```python
from build123d import *

# Parameters (mm, degrees)
F1_DEPTH = 19.05
F2_W     = 128.431639
F2_H     = 61.237093
F3_DEPTH = 6.35
F4_R     = 15.24


with BuildPart() as f1:
    # F0 (on Top) → F1 (new body)
    with BuildSketch(Plane.XY):
        Polygon((-110.641599, 45.212001), (-110.641599, -23.367999), (26.518401, -23.367999), (26.518401, -16.519178), (-99.390604, -16.519178), (-99.390604, 38.352568), (26.518401, 38.352568), (26.518401, 45.212001), align=None)
    extrude(amount=F1_DEPTH)

    # F2 (on Top) → F3 (join)
    with BuildSketch(Plane.XY):
        with Locations((-37.725527, 10.113819)):
            Rectangle(F2_W, F2_H)
    extrude(amount=F3_DEPTH)

    # F4
    f4_edges = [f1.edges().sort_by_distance(p)[0] for p in [
        (-110.641599, 10.922001, 0),
    ]]
    fillet(f4_edges, radius=F4_R)


solid = f1.part
```
Part model, mm, in its own coordinate system. A direction names the side the tool comes from. Give positions to 0.01 mm unless a question says otherwise; leave off trailing zeros. Order: outer loops, then holes, each group sorted by start corner. A loop starts at its lowest first (then second) coordinate and runs counter-clockwise, first axis right, second up. Notation, with made-up numbers: (4.5, 39.25) - (37.5, 39.25) arc R20 ccw to (37.5, 78.25) - close; hole circle Ø5 at (-22, 71). An arc over 180 degrees is marked (long way). Use one line per item in the form item = value.
Item 1: Which spindle directions (+Z, -Z, +X, -X, +Y, -Y) get a long thin tool onto all of the face, cutting with end or side? Do faces 1 (the face through (26.518, 42, 9)), 2 (the face through (-99.391, 11, 13)). Say none if no direction does.
Solution:
face_1 = +Z, -Z, +X, +Y, -Y
face_2 = +Z, +X
Item 2: Pin check, flat tips, straight feed: pin 1 Ø5 at (y, z) = (4, 1.5) entering from +X; pin 2 Ø12 at (x, y) = (-36.5, 6) entering from +Z; pin 3 Ø10 at (y, z) = (8.5, 13) entering from +X. Stop position of each tip, or through.
Solution:
pin_1 = 26.49
pin_2 = 6.35
pin_3 = -99.39
Item 3: Slice it at A-A on x = -50.5. Give the cut face in (y, z).
Solution:
outline = (-23.37, 0) - (45.21, 0) - (45.21, 19.05) - (38.35, 19.05) - (38.35, 6.35) - (-16.52, 6.35) - (-16.52, 19.05) - (-23.37, 19.05) - close
Item 4: Probe probe 1 along Y at (x, z) = (19, 16.25); probe 2 along Z at (x, y) = (7.5, -1); probe 3 along X at (y, z) = (-2, 16). List the from-to ranges inside material, lowest first. Write a range as from..to.
Solution:
probe_1 = -23.37..-16.52, 38.35..45.21
probe_2 = 0..6.35
probe_3 = -110.64..-99.39
Item 5: Slice it at D-D on y = 22. Give the cut face in (x, z), and give its area (3 significant figures).
Solution:
outline = (-110.64, 15.24) arc R15.24 ccw to (-95.4, 0) - (26.49, 0) - (26.49, 6.35) - (-99.39, 6.35) - (-99.39, 19.05) - (-110.64, 19.05) - close
area = 964 mm2
Item 6: Two-plate mould, pull along Y, no slides. Class faces 3 (the face through (-110.642, 11, 17)), 4 (the face through (-43, -23.368, 9)), 5 (the face through (-37, 38.353, 14)): released by +Y, released by -Y, zero draft, split by the parting line, or undercut.
Solution:
face_3 = zero draft
face_4 = released by -Y
face_5 = undercut
Item 7: Slice it at B-B on y = -18.5. Give the cut face in (x, z).
Solution:
outline = (-110.64, 15.24) arc R15.24 ccw to (-95.4, 0) - (26.52, 0) - (26.52, 19.05) - (-110.64, 19.05) - close
